Design review of the part built by this model. Coordinates are the model's own, in mm. Round coordinates to 2 decimals unless told otherwise and drop trailing zeros. Order: outer loops, then holes, each group sorted by start corner. A loop starts at its lowest first (then second) coordinate and runs counter-clockwise, first axis right, second up. Notation, with made-up numbers: M 30.25,68 L 62.25,68 A15 ccw 62.25,81 Z; hole C 30,-3 d11. An arc over 180 degrees is marked long. Use a Markdown table: item, result. Add a question column.
(1) For pin 1 (3.5 mm diameter, centred on x = 5.69, y = -17.96, fed in from +Z); pin 2 (3 mm diameter, centred on x = -26.5, z = 9.5, fed in from +Y); pin 3 (5 mm diameter, centred on x = 13.5, z = 10.5, fed in from -Y), all flat-tipped, find the tip position at first contact; note any pin that passes through.
(2) The part is to be moulded in two halves that separate along X. For faces 1 (the face through (-17.51, 6.3, 5.92)), 2 (the face through (-25.236, -32.516, 5.916)), 3 (the face through (21.335, -6, 6)), say which applies: released by +X, released by -X, zero draft, split by the parting line, or undercut.
(3) To check wall thickness, follow probe 1 along Y at (x, z) = (5.5, 5.75); probe 2 along X at (y, z) = (-22.5, 6.5); probe 3 along X at (y, z) = (-22, 2). State the ranges of each line that lie inside material, in increasing order. Write a range as from..to.
(4) Take a section at B-B (x = -7.5). Write out the cut boundary in (y, z), then the cut area to 3 significant figures.
(5) Take a section at C-C (x = 5). Write out the cut boundary in (y, z), then the cut area to 3 significant figures.
(6) Take a section at A-A (y = -2). Write out the cut boundary in (x, z), then the cut area to 3 significant figures.
(7) Take a section at D-D (z = 9). Count the separate pieces of the cut face and the enclosed holes in it, then the cut area to 3 significant figures.
Autodesk Inventor part; units mm, degrees
ref_plane "YZ Plane" through (0, 0, 0) normal (1, 0, 0) x (0, 1, 0)
ref_plane "XZ Plane" through (0, 0, 0) normal (0, 1, 0) x (-1, 0, 0)
ref_plane "XY Plane" through (0, 0, 0) normal (0, 0, 1) x (1, 0, 0)
sketch "Base" plane through (0, 0, 0) normal (0, 0, 1) x (1, 0, 0)
  circle A0 centre (18.3354, -21.8597) radius 1.2295
  circle A1 centre (-31.6646, -21.8597) radius 1.2295
  circle A2 centre (18.3354, 10.6981) radius 1.2295
  circle A3 centre (-31.6646, 10.6981) radius 1.2295
  circle A4 centre (-6.6646, -5.5808) radius 5
  arc A5 (21.3354, 10.6981) -> (17.758, 13.642) centre (18.3354, 10.6981) ccw
  arc A6 (12.5583, 18.8418) -> (17.758, 13.642) centre (16.9054, 17.9892) ccw
  arc A7 (12.5583, 18.8418) -> (9.6143, 22.4192) centre (9.6143, 19.4192) ccw
  line L0 (9.6143, 22.4192) -> (-22.9435, 22.4192)
  arc A8 (-22.9435, 22.4192) -> (-25.8874, 18.8418) centre (-22.9435, 19.4192) ccw
  arc A9 (-31.0872, 13.642) -> (-25.8874, 18.8418) centre (-30.2346, 17.9892) ccw
  arc A10 (-31.0872, 13.642) -> (-34.6646, 10.6981) centre (-31.6646, 10.6981) ccw
  line L1 (-34.6646, 10.6981) -> (-34.6646, -21.8597)
  arc A11 (-34.6646, -21.8597) -> (-31.0872, -24.8036) centre (-31.6646, -21.8597) ccw
  arc A12 (-25.8874, -30.0034) -> (-31.0872, -24.8036) centre (-30.2346, -29.1508) ccw
  arc A13 (-25.8874, -30.0034) -> (-22.9435, -33.5808) centre (-22.9435, -30.5808) ccw
  line L2 (-22.9435, -33.5808) -> (9.6143, -33.5808)
  arc A14 (9.6143, -33.5808) -> (12.5583, -30.0034) centre (9.6143, -30.5808) ccw
  arc A15 (17.758, -24.8036) -> (12.5583, -30.0034) centre (16.9054, -29.1508) ccw
  arc A16 (17.758, -24.8036) -> (21.3354, -21.8597) centre (18.3354, -21.8597) ccw
  line L3 (21.3354, -21.8597) -> (21.3354, 10.6981)
  circle A17 centre (-19.0581, -17.9611) radius 1.6234
  circle A18 centre (-19.0582, 6.7882) radius 1.6241
  circle A19 centre (5.6908, 6.7877) radius 1.6234
  circle A20 centre (5.6907, -17.9611) radius 1.6235
  point P0 (0, 0)
extrude "Plate1" add sketch "Base" along normal blind 12
equation "\"d0\" = Thickness"
equation "\"BendRadius\" = Thickness"
equation "\"BendReliefWidth\" = Thickness"
equation "\"BendReliefDepth\" = 0.5 * Thickness"
equation "\"CornerReliefSize\" = 4 * Thickness"
equation "\"MinimumRemnant\" = 2 * Thickness"
equation "\"TransitionRadius\" = BendRadius"
equation "\"JacobiRadiusSize\" = BendRadius"
equation "\"GapSize\" = Thickness"
properties part number "NeckEncoderMount"
Verdict:
| question | item | result |
|---|---|---|
| 1 | pin 1 | stops at z = 12 |
| 1 | pin 2 | stops at y = 21.6 |
| 1 | pin 3 | stops at y = -33.24 |
| 2 | face 1 | undercut |
| 2 | face 2 | released by -X |
| 2 | face 3 | released by +X |
| 3 | probe 1 | y = -33.58..-19.57, -16.35..5.18, 8.4..22.42 |
| 3 | probe 2 | x = -34.6..-32.71, -30.61..17.29, 19.39..21.27 |
| 3 | probe 3 | x = -34.66..-32.89, -30.44..17.11, 19.56..21.33 |
| 4 | outline | M -33.58,0 L -10.51,0 L -10.51,12 L -33.58,12 Z; M -0.65,0 L 22.42,0 L 22.42,12 L -0.65,12 Z |
| 4 | area | 554 mm^2 |
| 5 | outline | M -33.58,0 L -19.43,0 L -19.43,12 L -33.58,12 Z; M -16.49,0 L 5.32,0 L 5.32,12 L -16.49,12 Z; M 8.26,0 L 22.42,0 L 22.42,12 L 8.26,12 Z |
| 5 | area | 601 mm^2 |
| 6 | outline | M -34.66,0 L -10.15,0 L -10.15,12 L -34.66,12 Z; M -3.17,0 L 21.34,0 L 21.34,12 L -3.17,12 Z |
| 6 | area | 588 mm^2 |
| 7 | separate pieces | 1 |
| 7 | enclosed holes | 9 |
| 7 | area | 2,700 mm^2 |
